```python
from build123d import *

# Parameters (mm, degrees)
F0_W           = 105
F0_H           = 85
F0_R           = 4
F1_DEPTH       = 8
F2_D           = 8.8
F2_CBORE_D     = 14.25
F2_CBORE_DEPTH = 8


with BuildPart() as f1:
    # F0 (on Top) → F1 (new body)
    with BuildSketch(Plane.XY):
        Rectangle(F0_W, F0_H)
        with Locations((-40, -30)):
            Circle(F0_R, mode=Mode.SUBTRACT)
        with Locations((40, -30)):
            Circle(F0_R, mode=Mode.SUBTRACT)
        with Locations((-40, 30)):
            Circle(F0_R, mode=Mode.SUBTRACT)
        with Locations((40, 30)):
            Circle(F0_R, mode=Mode.SUBTRACT)
        with Locations((-40, 30)):
            Circle(F0_R)
        with Locations((40, 30)):
            Circle(F0_R)
        with Locations((40, -30)):
            Circle(F0_R)
        with Locations((-40, -30)):
            Circle(F0_R)
    extrude(amount=F1_DEPTH)

    # F2 (through all)
    with Locations(Plane(origin=(0, 0, 0), x_dir=(1, 0, 0), z_dir=(0, 0, -1))):
        with Locations((-40, -30), (40, -30), (40, 30), (-40, 30)):
            CounterBoreHole(F2_D / 2, F2_CBORE_D / 2, F2_CBORE_DEPTH)


solid = f1.part
```
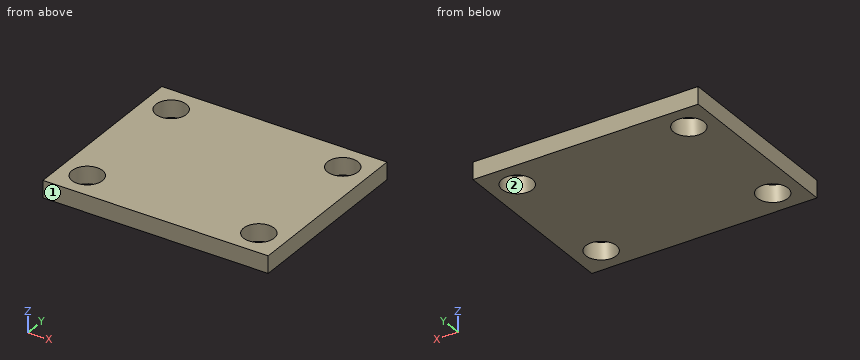
Part model, mm, in its own coordinate system. Face numbers are marked on the shaded views. Coordinates: 2 decimals unless noted, no trailing zeros. Order: outer loops, then holes, each group sorted by start corner. A loop starts at its lowest first (then second) coordinate and runs counter-clockwise, first axis right, second up. Notation, with made-up numbers: (-3.75, 31) - (50.25, 31) arc R14 cw to (50.25, 43) - close; hole circle Ø4 at (20.25, 32). An arc over 180 degrees is marked (long way). Return JSON: item names as keys, results as strings. Group by question number.
Item 1: Cut at B-B (x = 40). List the corners of the cut face in (y, z) (3 decimals), plus the area to 3 significant figures.
Item 2: Pull direction X, two halves, no side cores. Call the marked faces 1 and 2: pulls with the +X half, pulls with the -X half, needs draft (parallel to the pull), parting line crosses it, or undercut.
Item 3: Drill centre lines: probe 1 along Y at (x, z) = (-40, 6) (3 decimals); probe 2 along X at (y, z) = (-30, 6) (3 decimals); probe 3 along X at (y, z) = (-35, 2). Where is each one in solid material? Low to high. Write a range as from..to.
Item 4: Cut at A-A (y = 30). List the corners of the cut face in (x, z) (3 decimals).
Item 5: Pin check, flat tip, straight feed: pin 1 (8.5 mm diameter, centred on x = -40, y = -30, fed in from +Z). Stop position of the tip, or through.
Item 6: Cut at C-C (z = 2.75). List the corners of the cut face in (x, y) (3 decimals).
Check values:
{
 "1": {"outline": "(-42.5, 0) - (-37.125, 0) - (-37.125, 8) - (-42.5, 8) - close; (-22.875, 0) - (22.875, 0) - (22.875, 8) - (-22.875, 8) - close; (37.125, 0) - (42.5, 0) - (42.5, 8) - (37.125, 8) - close", "area": "452 mm2"},
 "2": {"face 1": "needs draft", "face 2": "undercut"},
 "3": {"probe 1": "y = -42.5..-37.125, -22.875..22.875, 37.125..42.5", "probe 2": "x = -52.5..-47.125, -32.875..32.875, 47.125..52.5", "probe 3": "x = -52.5..-45.08, -34.92..34.92, 45.08..52.5"},
 "4": {"outline": "(-52.5, 0) - (-47.125, 0) - (-47.125, 8) - (-52.5, 8) - close; (-32.875, 0) - (32.875, 0) - (32.875, 8) - (-32.875, 8) - close; (47.125, 0) - (52.5, 0) - (52.5, 8) - (47.125, 8) - close"},
 "5": {"pin 1": "passes through"},
 "6": {"outline": "(-52.5, -42.5) - (52.5, -42.5) - (52.5, 42.5) - (-52.5, 42.5) - close; hole circle Ø14.25 at (-40, -30); hole circle Ø14.25 at (-40, 30); hole circle Ø14.25 at (40, -30); hole circle Ø14.25 at (40, 30)"}
}
